Source: CAD feature listing. Evaluate the final solid. Frame: model axes, mm. Face numbers are marked on the shaded views. A direction names the side the tool comes from. Coordinates: 2 decimals unless noted, no trailing zeros. Loops run counter-clockwise (first coordinate to the right, second up) from the corner with the lowest first, then second, coordinate; pieces in that order, holes last.
Item 1: Section query C-C, the plane z = -8. Return the cut outline in (x, y).
Item 2: Reachability of the marked faces 1 and 2 from +Z, -Z, +X, -X, +Y, -Y: full face, straight path, thin tool, end or side. Return the list, or none.
Item 3: Section query B-B, the plane y = -39.5. Return the cut outline in (x, z), then the cut area to 3 significant figures.
Item 4: Line query: probe 1 along Y at (x, z) = (15.5, -30); probe 2 along X at (y, z) = (-30, -4.5). Output: solid intervals per line, ascending.
Item 5: Section query D-D, the plane z = -15.5. Return the cut outline in (x, y), then the cut area to 3 significant figures.
Item 6: Pin query (flat end, axial travel): pin 1 Ø10 at (x, z) = (17.5, -13.5) entering from +Y; pin 2 Ø6 at (y, z) = (-22, -31.5) entering from +X. Return the tip coordinate at first contact, or that it passes through.
Item 7: Section query A-A, the plane z = -24. Return the cut outline in (x, y), then the cut area to 3 significant figures.
```python
from build123d import *

# Parameters (mm, degrees)
BOSS_EXTRUDE1_DEPTH = 40
FILLET1_R           = 20
FILLET2_R           = 20
SKETCH2_R           = 6
CUT_EXTRUDE1_DEPTH  = 10


with BuildPart() as part:
    # Sketch1 → Boss-Extrude1 (new body)
    with BuildSketch(Plane.XY):
        Polygon((0, 0), (0, -45), (45, -45), (45, -43), (2, -43), (2, 0), align=None)
    extrude(amount=-BOSS_EXTRUDE1_DEPTH)

    # Fillet1
    fillet1_edges = [part.edges().sort_by_distance(p)[0] for p in [
        (1, 0, -40),
    ]]
    fillet(fillet1_edges, radius=FILLET1_R)

    # Fillet2
    fillet2_edges = [part.edges().sort_by_distance(p)[0] for p in [
        (1, 0, 0),
    ]]
    fillet(fillet2_edges, radius=FILLET2_R - 0.0001)  # a hair under: the kernel refuses the full size

    # Sketch2 → Cut-Extrude1 (cut)
    with BuildSketch(Plane.ZY):
        with Locations(Location((-20, -13.002174514, 0), (0, 0, 270))):
            Circle(SKETCH2_R)
    extrude(amount=-CUT_EXTRUDE1_DEPTH, mode=Mode.SUBTRACT)


solid = part.part
```
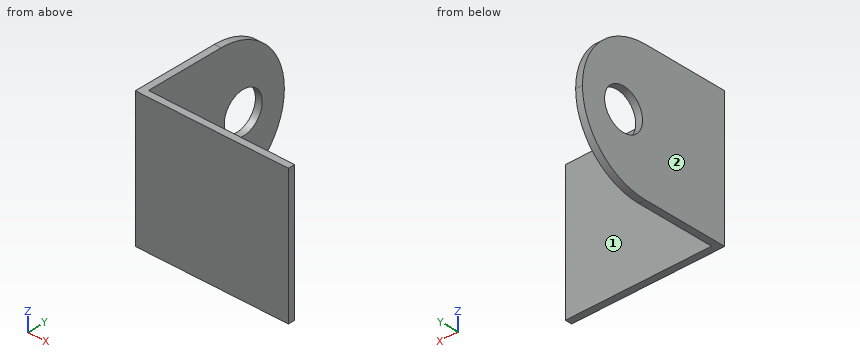
Verdict:
1. outline: (0, -45) - (45, -45) - (45, -43) - (2, -43) - (2, -4) - (0, -4) - close
2. face 1: +Z, -Z, +X, +Y
2. face 2: +Z, -Z, -X, +Y, -Y
3. outline: (0, -40) - (2, -40) - (2, 0) - (0, 0) - close
3. area: 80.0 mm2
4. probe 1: y = -45 to -43
4. probe 2: x = 0 to 2
5. outline: (0, -45) - (45, -45) - (45, -43) - (2, -43) - (2, -16.97) - (0, -16.97) - close; (0, -9.03) - (2, -9.03) - (2, -0.51) - (0, -0.51) - close
5. area: 159 mm2
6. pin 1: stops at y = -43
6. pin 2: stops at x = 2
7. outline: (0, -45) - (45, -45) - (45, -43) - (2, -43) - (2, -17.47) - (0, -17.47) - close; (0, -8.53) - (2, -8.53) - (2, -0.4) - (0, -0.4) - close
7. area: 157 mm2
